```python
from build123d import *

# Parameters (mm, degrees)
SKETCH1_R           = 2.5
BOSS_EXTRUDE1_DEPTH = 354


with BuildPart() as part:
    # Sketch1 → Boss-Extrude1 (new body)
    with BuildSketch(Plane.XY):
        with BuildLine():
            Line((2.839339828, 3.9), (-2.839339828, 3.9))
            Line((-2.839339828, 3.9), (-5.5, 6.560660172))
            Line((-5.5, 6.560660172), (-5.5, 8.2))
            Line((-5.5, 8.2), (-3.1, 8.2))
            Line((-3.1, 8.2), (-3.1, 9))
            Line((-3.1, 9), (-4.1, 10))
            Line((-4.1, 10), (-8.5, 10))
            ThreePointArc((-8.5, 10), (-9.560660172, 9.560660172), (-10, 8.5))
            Line((-10, 8.5), (-10, 4.1))
            Line((-10, 4.1), (-9, 3.1))
            Line((-9, 3.1), (-8.2, 3.1))
            Line((-8.2, 3.1), (-8.2, 5.5))
            Line((-8.2, 5.5), (-6.560660172, 5.5))
            Line((-6.560660172, 5.5), (-3.9, 2.839339828))
            Line((-3.9, 2.839339828), (-3.9, -2.839339828))
            Line((-3.9, -2.839339828), (-6.560660172, -5.5))
            Line((-6.560660172, -5.5), (-8.2, -5.5))
            Line((-8.2, -5.5), (-8.2, -3.1))
            Line((-8.2, -3.1), (-9, -3.1))
            Line((-9, -3.1), (-10, -4.1))
            Line((-10, -4.1), (-10, -8.5))
            ThreePointArc((-10, -8.5), (-9.560660172, -9.560660172), (-8.5, -10))
            Line((-8.5, -10), (-4.1, -10))
            Line((-4.1, -10), (-3.1, -9))
            Line((-3.1, -9), (-3.1, -8.2))
            Line((-3.1, -8.2), (-5.5, -8.2))
            Line((-5.5, -8.2), (-5.5, -6.560660172))
            Line((-5.5, -6.560660172), (-2.839339828, -3.9))
            Line((-2.839339828, -3.9), (2.839339828, -3.9))
            Line((2.839339828, -3.9), (5.5, -6.560660172))
            Line((5.5, -6.560660172), (5.5, -8.2))
            Line((5.5, -8.2), (3.1, -8.2))
            Line((3.1, -8.2), (3.1, -9))
            Line((3.1, -9), (4.1, -10))
            Line((4.1, -10), (8.5, -10))
            ThreePointArc((8.5, -10), (9.560660172, -9.560660172), (10, -8.5))
            Line((10, -8.5), (10, -4.1))
            Line((10, -4.1), (9, -3.1))
            Line((9, -3.1), (8.2, -3.1))
            Line((8.2, -3.1), (8.2, -5.5))
            Line((8.2, -5.5), (6.560660172, -5.5))
            Line((6.560660172, -5.5), (3.9, -2.839339828))
            Line((3.9, -2.839339828), (3.9, 2.839339828))
            Line((3.9, 2.839339828), (6.560660172, 5.5))
            Line((6.560660172, 5.5), (8.2, 5.5))
            Line((8.2, 5.5), (8.2, 3.1))
            Line((8.2, 3.1), (9, 3.1))
            Line((9, 3.1), (10, 4.1))
            Line((10, 4.1), (10, 8.5))
            ThreePointArc((10, 8.5), (9.560660172, 9.560660172), (8.5, 10))
            Line((8.5, 10), (4.1, 10))
            Line((4.1, 10), (3.1, 9))
            Line((3.1, 9), (3.1, 8.2))
            Line((3.1, 8.2), (5.5, 8.2))
            Line((5.5, 8.2), (5.5, 6.560660172))
            Line((5.5, 6.560660172), (2.839339828, 3.9))
        make_face()
        Circle(SKETCH1_R, mode=Mode.SUBTRACT)
    extrude(amount=BOSS_EXTRUDE1_DEPTH)


solid = part.part
```
Verification items for the finished model (mm, model axes). A direction names the side the tool comes from. Coordinates: 2 decimals unless noted, no trailing zeros. Return JSON: item names as keys, results as strings.
1. Thickness scan on L1, parallel to Y at x = 0, z = 73.5; L2, parallel to X at y = -0.5, z = 180; L3, parallel to X at y = 4.25, z = 211. Record the ranges inside material, lowest first.
Established:
{"L1": "y = -3.9 to -2.5, 2.5 to 3.9", "L2": "x = -3.9 to -2.45, 2.45 to 3.9", "L3": "x = -10 to -8.2, -5.31 to -3.19, 3.19 to 5.31, 8.2 to 10"}
2. Go/stop test with a flat-tipped pin: pin 1 (4 mm diameter, centred on x = 4, z = 73.5, fed in from -Y). Record where the tip stops, or that it passes through.
Established:
{"pin 1": "stops at y = -10"}
3. Tool access check on faces 4 (the flat face through (-3.9, 0, 175)), 5 (the flat face through (0, 3.9, 175)), 6 (the flat face through (2, 2, 0)). Record the directions out of +Z, -Z, +X, -X, +Y, -Y that give a thin tool (end or side, any length) a straight path to the whole face; none if there is none.
Established:
{"face 4": "+Z, -Z, -X", "face 5": "+Z, -Z, +Y", "face 6": "-Z, +X, -X, +Y, -Y"}
4. Mould release check, pull along X, two halves, no side actions. Record for faces 1 (the flat face through (3.9, 0, 175)), 2 (the flat face through (2, 2, 354)), 3 (the flat face through (0, -3.9, 175)): +X half, -X half, draft (parallel to the pull), parting line (faces both ways), or undercut.
Established:
{"face 1": "+X half", "face 2": "draft", "face 3": "undercut"}
